```python
from build123d import *

# Parameters (mm, degrees)
SKETCH1_R           = 2.032
BOSS_EXTRUDE1_DEPTH = 6.35


with BuildPart() as part:
    # Sketch1 → Boss-Extrude1 (new body)
    with BuildSketch(Plane.XY):
        Polygon((69.85, 0), (88.9, 38.1), (88.9, 50.8), (0, 50.8), (0, 0), align=None)
        with Locations((6.35, 6.35)):
            Circle(SKETCH1_R, mode=Mode.SUBTRACT)
        with Locations((19.05, 6.35)):
            Circle(SKETCH1_R, mode=Mode.SUBTRACT)
        with Locations((19.05, 44.45)):
            Circle(SKETCH1_R, mode=Mode.SUBTRACT)
        with Locations((6.35, 44.45)):
            Circle(SKETCH1_R, mode=Mode.SUBTRACT)
        with Locations((12.7, 25.4)):
            Circle(SKETCH1_R, mode=Mode.SUBTRACT)
    extrude(amount=BOSS_EXTRUDE1_DEPTH)


solid = part.part
```
Input: part model. Units: mm. Frame: model coordinates. Round coordinates to 2 decimals unless told otherwise and drop trailing zeros. Loops run counter-clockwise (first coordinate to the right, second up) from the corner with the lowest first, then second, coordinate; pieces in that order, holes last. Notation, with made-up numbers: (-25.75, 2.25) -> (-3.75, 2.25) arc R16 ccw to (-3.75, 14.25) -> close; hole circle Ø5 at (-39.5, 1). An arc over 180 degrees is marked (long way). Use one line per item in the form item = value. Start each with the question number.
Item 1: Section query C-C on z = 2.5. Return the cut outline in (x, y).
Item 2: Mould query, pull axis Y, two halves, no side actions, for faces 1 (the face through (45, 50.8, 3)), 2 (the face through (17.44, 43.21, 3.13)), 3 (the face through (79.24, 18.78, 3.13)). Classes: pulls with the +Y half, pulls with the -Y half, needs draft (parallel to the pull), parting line crosses it, or undercut.
Item 3: Contact query for a flat-ended pin moving along its axis: pin 1 Ø3.5 at (x, y) = (19.05, 44.45) entering from +Z. Output: stop coordinate, or through.
Item 4: Section query B-B on y = 44.45. Return the cut outline in (x, z).
Item 5: Material intervals for L1, parallel to Y at x = 6.35, z = 5; L2, parallel to Y at x = 7, z = 4; L3, parallel to X at y = 8, z = 6, sorted ascending. Write a range as from..to.
Item 6: Section query A-A on x = 6.35. Return the cut outline in (y, z).
Item 7: Section query D-D on y = 25.4. Return the cut outline in (x, z).
Ans:
q1.outline = (0, 0) -> (69.85, 0) -> (88.9, 38.1) -> (88.9, 50.8) -> (0, 50.8) -> close; hole circle Ø4.06 at (6.35, 6.35); hole circle Ø4.06 at (6.35, 44.45); hole circle Ø4.06 at (12.7, 25.4); hole circle Ø4.06 at (19.05, 6.35); hole circle Ø4.06 at (19.05, 44.45)
q2.face_1 = pulls with the +Y half
q2.face_2 = undercut
q2.face_3 = pulls with the -Y half
q3.pin_1 = through
q4.outline = (0, 0) -> (4.32, 0) -> (4.32, 6.35) -> (0, 6.35) -> close; (8.38, 0) -> (17.02, 0) -> (17.02, 6.35) -> (8.38, 6.35) -> close; (21.08, 0) -> (88.9, 0) -> (88.9, 6.35) -> (21.08, 6.35) -> close
q5.L1 = 0..4.32, 8.38..42.42, 46.48..50.8
q5.L2 = 0..4.42, 8.28..42.52, 46.38..50.8
q5.L3 = 0..5.16, 7.54..17.86, 20.24..73.85
q6.outline = (0, 0) -> (4.32, 0) -> (4.32, 6.35) -> (0, 6.35) -> close; (8.38, 0) -> (42.42, 0) -> (42.42, 6.35) -> (8.38, 6.35) -> close; (46.48, 0) -> (50.8, 0) -> (50.8, 6.35) -> (46.48, 6.35) -> close
q7.outline = (0, 0) -> (10.67, 0) -> (10.67, 6.35) -> (0, 6.35) -> close; (14.73, 0) -> (82.55, 0) -> (82.55, 6.35) -> (14.73, 6.35) -> close
